```python
from build123d import *

# Parameters (mm, degrees)
F0_R     = 1.7272
F1_DEPTH = 3.175
F2_R     = 0.762


with BuildPart() as f1:
    # F0 (on Top) → F1 (new body)
    with BuildSketch(Plane.XY):
        with BuildLine():
            Line((-25.750805, -73.88963), (43.790972, -73.88963))
            Line((43.790972, -73.88963), (43.790972, 73.88963))
            Line((43.790972, 73.88963), (26.324776, 73.88963))
            ThreePointArc((26.324776, 73.88963), (20.730742, 71.525126), (18.528473, 65.865257))
            Line((18.528473, 65.865257), (18.82983, 55.415228))
            Line((18.82983, 55.415228), (0.468945, 37.308589))
            ThreePointArc((0.468945, 37.308589), (-0.687524, 32.359758), (3.280937, 29.184909))
            ThreePointArc((3.280937, 29.184909), (26.003765, -13.65019), (-22.15767, -19.275922))
            ThreePointArc((-22.15767, -19.275922), (-27.419502, -17.941157), (-30.513305, -22.401747))
            Line((-30.513305, -22.401747), (-30.513305, -43.822152))
            ThreePointArc((-30.513305, -43.822152), (-7.010584, -50.526938), (-30.513305, -57.231725))
            Line((-30.513305, -57.231725), (-30.513305, -69.12713))
            ThreePointArc((-30.513305, -69.12713), (-29.118401, -72.494726), (-25.750805, -73.88963))
        make_face()
        with Locations((-25.750805, -69.12713)):
            Circle(F0_R, mode=Mode.SUBTRACT)
        with Locations((-16.225805, -69.12713)):
            Circle(F0_R, mode=Mode.SUBTRACT)
        with Locations((1.046195, -69.12713)):
            Circle(F0_R, mode=Mode.SUBTRACT)
        with Locations((-25.750805, -31.926747)):
            Circle(F0_R, mode=Mode.SUBTRACT)
        with Locations((-25.750805, -22.401747)):
            Circle(F0_R, mode=Mode.SUBTRACT)
        with Locations((39.028472, -58.64963)):
            Circle(F0_R, mode=Mode.SUBTRACT)
        with Locations((39.028472, -39.59963)):
            Circle(F0_R, mode=Mode.SUBTRACT)
        with Locations((3.812981, 33.917597)):
            Circle(F0_R, mode=Mode.SUBTRACT)
        with Locations((39.028472, 39.59963)):
            Circle(F0_R, mode=Mode.SUBTRACT)
        with Locations((39.028472, 58.64963)):
            Circle(F0_R, mode=Mode.SUBTRACT)
    extrude(amount=F1_DEPTH)

    # F2
    f2_edges = [f1.edges().sort_by_distance(p)[0] for p in [
        (-30.513305, -43.822152, 1.5875),
        (-30.513305, -57.231725, 1.5875),
    ]]
    fillet(f2_edges, radius=F2_R)


solid = f1.part
```
The model under review builds one solid part; all positions refer to its coordinate system, in mm. Round coordinates to 2 decimals unless told otherwise and drop trailing zeros. Loops run counter-clockwise (first coordinate to the right, second up) from the corner with the lowest first, then second, coordinate; pieces in that order, holes last. Notation, with made-up numbers: (53.5, 68.25) - (74.5, 68.25) arc R5 ccw to (74.5, 73.25) - close; hole circle Ø3 at (-6.75, 88.25). An arc over 180 degrees is marked (long way). Use a Markdown table: item, result. Add a question column.
Q1. Add section A-A (x = 22). State the section outline as (y, z) points (3 decimals).
Q2. Add section D-D (x = -5). State the section outline as (y, z) points (3 decimals).
Q3. Add section C-C (y = 0). State the section outline as (x, z) points (3 decimals).
Q4. The part is to be moulded in two halves that separate along X. For faces 1 (the face through (38.804, -37.887, 1.565)), 2 (the face through (9, -73.89, 2)), 3 (the face through (-29.155, -72.457, 1.565)), 4 (the face through (43.791, -1, 2)), say which applies: pulls with the +X half, pulls with the -X half, needs draft (parallel to the pull), parting line crosses it, or undercut.
Q5. Add section B-B (z = 2.3). State how many separate pieces and enclosed holes the cut face has, plus the area to 3 significant figures.
Q6. For probe 1 along X at (y, z) = (34, 0.4); probe 2 along Y at (x, z) = (4, 2.1); probe 3 along Y at (x, z) = (2, 0.5), list the stretches that pass through material, from the lowest coordinate up.
Q7. Insertion check: pin 1 Ø4.5 at (x, y) = (1.05, -69.13) entering from -Z; pin 2 Ø12 at (x, y) = (-6, 21.5) entering from +Z. Each pin has a flat end and moves straight along its axis. Give the tip position at first contact, or say it passes through.
Worked answers:
| question | item | result |
|---|---|---|
| 1 | outline | (-73.89, 0) - (-19.456, 0) - (-19.456, 3.175) - (-73.89, 3.175) - close; (19.456, 0) - (72.581, 0) - (72.581, 3.175) - (19.456, 3.175) - close |
| 2 | outline | (-73.89, 0) - (-28.94, 0) - (-28.94, 3.175) - (-73.89, 3.175) - close |
| 3 | outline | (29.369, 0) - (43.791, 0) - (43.791, 3.175) - (29.369, 3.175) - close |
| 4 | face 1 | undercut |
| 4 | face 2 | needs draft |
| 4 | face 3 | pulls with the -X half |
| 4 | face 4 | pulls with the +X half |
| 5 | separate pieces | 1 |
| 5 | enclosed holes | 10 |
| 5 | area | 5,510 mm² |
| 6 | probe 1 | -0.95 to 2.09, 5.54 to 43.79 |
| 6 | probe 2 | -73.89 to -29.1, 29.1 to 32.2, 35.63 to 40.79 |
| 6 | probe 3 | -73.89 to -70.57, -67.69 to -29.3, 29.51 to 38.82 |
| 7 | pin 1 | z = 0 |
| 7 | pin 2 | through |
